Could you check a few things on this model? Use its own coordinates, in mm. Face numbers are marked on the shaded views. Give positions to 0.01 mm unless a question says otherwise; leave off trailing zeros. Loops run counter-clockwise (first coordinate to the right, second up) from the corner with the lowest first, then second, coordinate; pieces in that order, holes last. Notation, with made-up numbers: (-18, 28.5) -> (-6, 28.5) arc R13 ccw to (-6, 32.5) -> close; hole circle Ø9 at (-16.5, 9.5). An arc over 180 degrees is marked (long way). Put each result on its own line as item: value.
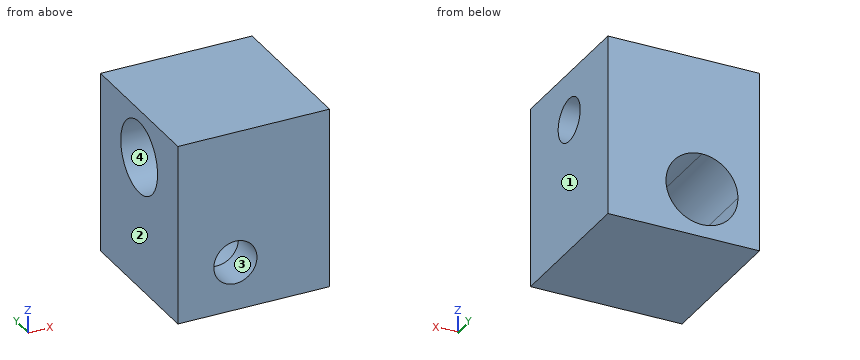
```python
from build123d import *

# Parameters (mm, degrees)
F0_W      = 12.00023
F0_H      = 10.0584
F1_DEPTH  = 24.00046
F2_W      = 24.00046
F2_H      = 37.6428
F3_DEPTH  = 7.62
F4_W      = 31.62046
F4_H      = 37.6428
F4_R      = 7.5057
F5_DEPTH  = 7.62
F6_R      = 4.5
F7_DEPTH  = 25.4
F9_DEPTH  = 24.00046
F10_R     = 4.5
F11_DEPTH = 25.4


with BuildPart() as f1:
    # F0 (on Front) → F1 (new body)
    with BuildSketch(Plane.XZ):
        with BuildLine():
            Line((0, 10.0584), (0, 0))
            Line((0, 0), (12.00023, 0))
            Line((12.00023, 0), (12.00023, 2.5527))
            ThreePointArc((12.00023, 2.5527), (6.6928986324, 4.7510686324), (4.49453, 10.0584))
            Line((4.49453, 10.0584), (0, 10.0584))
        make_face()
        with BuildLine():
            Line((0, 27.5844), (0, 10.0584))
            Line((0, 10.0584), (4.49453, 10.0584))
            ThreePointArc((4.49453, 10.0584), (6.6928986324, 15.3657313676), (12.00023, 17.5641))
            Line((12.00023, 17.5641), (12.00023, 27.5844))
            Line((12.00023, 27.5844), (0, 27.5844))
        make_face()
        with Locations((6.000115, 32.6136)):
            Rectangle(F0_W, F0_H)
        with Locations((18.000345, 32.6136)):
            Rectangle(F0_W, F0_H)
        with BuildLine():
            Line((19.50593, 10.0584), (24.00046, 10.0584))
            Line((24.00046, 10.0584), (24.00046, 27.5844))
            Line((24.00046, 27.5844), (12.00023, 27.5844))
            Line((12.00023, 27.5844), (12.00023, 17.5641))
            ThreePointArc((12.00023, 17.5641), (17.3075613676, 15.3657313676), (19.50593, 10.0584))
        make_face()
        with BuildLine():
            Line((12.00023, 2.5527), (12.00023, 0))
            Line((12.00023, 0), (24.00046, 0))
            Line((24.00046, 0), (24.00046, 10.0584))
            Line((24.00046, 10.0584), (19.50593, 10.0584))
            ThreePointArc((19.50593, 10.0584), (17.3075613676, 4.7510686324), (12.00023, 2.5527))
        make_face()
    extrude(amount=F1_DEPTH)

    # F2 (on face) → F3 (join)
    with BuildSketch(Plane.YZ.offset(24.00046)):
        with Locations((-12.00023, 18.8214)):
            Rectangle(F2_W, F2_H)
    extrude(amount=F3_DEPTH)

    # F4 (on face) → F5 (join)
    with BuildSketch(Plane.XZ.offset(24.00046)):
        with Locations((15.81023, 18.8214)):
            Rectangle(F4_W, F4_H)
        with Locations((12.00023, 10.0584)):
            Circle(F4_R, mode=Mode.SUBTRACT)
        with Locations((12.00023, 10.0584)):
            Circle(F4_R)
    extrude(amount=F5_DEPTH)

    # F6 (on face) → F7 (cut)
    with BuildSketch(Plane(origin=(0, -24.00046, 0), x_dir=(-1, 0, 0), z_dir=(0, 1, 0))):
        with Locations((-12.00023, 10.0584)):
            Circle(F6_R)
    extrude(amount=-F7_DEPTH, mode=Mode.SUBTRACT)

    # F8 (on face) → F9 (cut)
    with BuildSketch(Plane(origin=(0, 0, 0), x_dir=(0, -1, 0), z_dir=(-1, 0, 0))):
        with BuildLine():
            ThreePointArc((8.30453, 27.5971), (15.81023, 20.0914), (23.31593, 27.5971))
            Line((23.31593, 27.5971), (15.81023, 27.5971))
            Line((15.81023, 27.5971), (8.30453, 27.5971))
        make_face()
        with BuildLine():
            Line((15.81023, 27.5971), (23.31593, 27.5971))
            ThreePointArc((23.31593, 27.5971), (15.81023, 35.1028), (8.30453, 27.5971))
            Line((8.30453, 27.5971), (15.81023, 27.5971))
        make_face()
    extrude(amount=-F9_DEPTH, mode=Mode.SUBTRACT)

    # F10 (on face) → F11 (cut)
    with BuildSketch(Plane(origin=(24.00046, 0, 0), x_dir=(0, -1, 0), z_dir=(-1, 0, 0))):
        with Locations((15.81023, 27.5971)):
            Circle(F10_R)
    extrude(amount=-F11_DEPTH, mode=Mode.SUBTRACT)


solid = f1.part
```
1. I'm going to push a flat-ended pin straight in: pin 1 (14.5 mm diameter, centred on y = -15.81, z = 27.6, fed in from -X). Where does the tip first touch, or does it pass through?
Recorded:
pin 1: stops at x = 24
2. If we section it at C-C (z = 11): List the corners of the cut face in (x, y) for me, then the cut area to 3 significant figures.
Recorded:
outline: (0, -31.62) -> (7.6, -31.62) -> (7.6, -24) -> (4.55, -24) -> (4.55, 0) -> (0, 0) -> close; (16.4, -31.62) -> (31.62, -31.62) -> (31.62, 0) -> (19.45, 0) -> (19.45, -24) -> (16.4, -24) -> close
area: 575 mm^2
3. If we section it at A-A (x = 8.5): List the corners of the cut face in (y, z) for me.
Recorded:
outline: (-31.62, 0) -> (0, 0) -> (0, 3.42) -> (-24, 3.42) -> (-24, 7.23) -> (-31.62, 7.23) -> close; (-31.62, 12.89) -> (-24, 12.89) -> (-24, 16.7) -> (0, 16.7) -> (0, 37.64) -> (-31.62, 37.64) -> close; hole circle Ø15.01 at (-15.81, 27.6)
4. If we section it at B-B (y = -12): List the corners of the cut face in (x, z) for me, then the cut area to 3 significant figures.
Recorded:
outline: (0, 0) -> (31.62, 0) -> (31.62, 25.2) -> (24, 25.2) -> (24, 21.13) -> (0, 21.13) -> close; (0, 34.06) -> (24, 34.06) -> (24, 29.99) -> (31.62, 29.99) -> (31.62, 37.64) -> (0, 37.64) -> close; hole circle Ø15.01 at (12, 10.06)
area: 666 mm^2
5. If we section it at D-D (y = -28): List the corners of the cut face in (x, z) for me.
Recorded:
outline: (0, 0) -> (31.62, 0) -> (31.62, 37.64) -> (0, 37.64) -> close; hole circle Ø9 at (12, 10.06)
6. Thinking about a two-plate mould opening in X: for the marked faces 1, 2, 3 and 4, which applies, pulls with the +X half, pulls with the -X half, needs draft (parallel to the pull), parting line crosses it, or undercut?
Recorded:
face 1: pulls with the +X half
face 2: pulls with the -X half
face 3: undercut
face 4: needs draft
7. I need wall thicknesses on line 1 (Y direction, x = 10, z = 28); line 2 (Z direction, x = 11.5, y = -22.5); line 3 (Z direction, x = 12, y = -25). Which ranges of each line are inside material? Lowest first, please.
Recorded:
line 1: y = -31.62 to -23.31, -8.32 to 0
line 2: z = 0 to 2.57, 17.55 to 24.19, 31 to 37.64
line 3: z = 0 to 5.56, 14.56 to 37.64
